Input: dimensioned drawing with shaded views. Units: mm. Origin: part minimum x, y, z. A direction names the side the tool comes from. Give positions to 0.01 mm unless a question says otherwise; leave off trailing zeros. Order: outer loops, then holes, each group sorted by start corner. A loop starts at its lowest first (then second) coordinate and runs counter-clockwise, first axis right, second up.
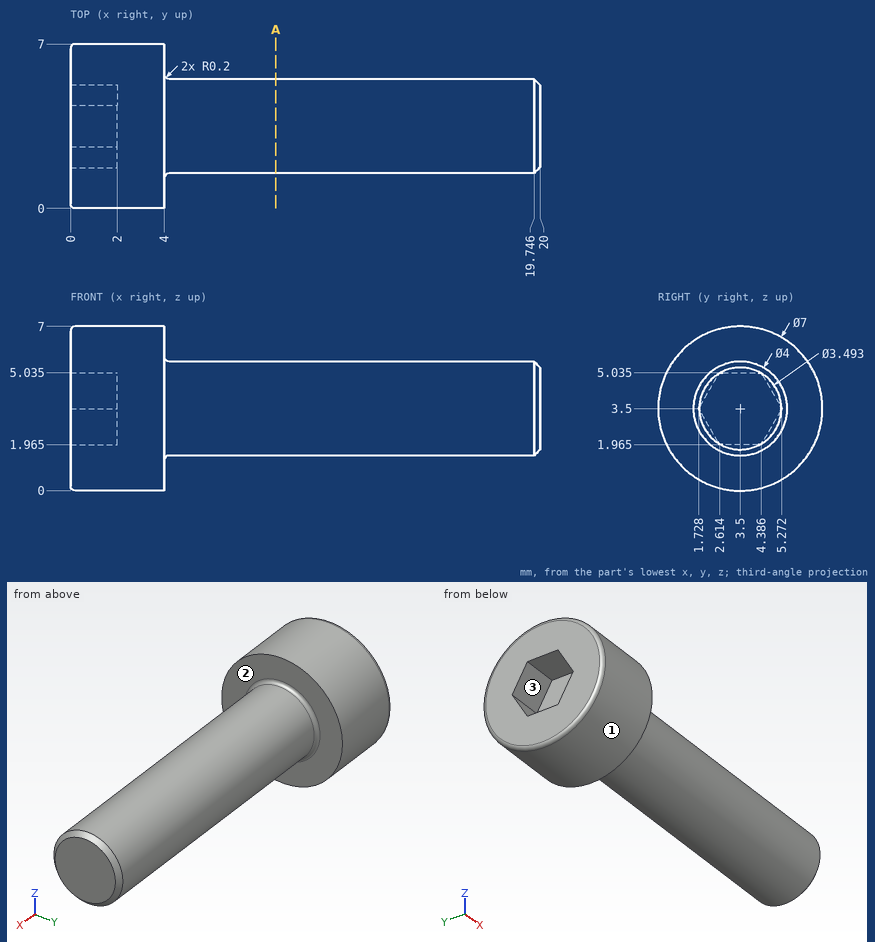
1) Pin query (flat end, axial travel): pin 1 (3 mm diameter, centred on x = 16.5, z = 6, fed in from -Y). Return the tip coordinate at first contact, or that it passes through.
Report:
pin 1: stops at y = 1.77
2) Section query A-A, the plane x = 8.75. Return the cut outline in (y, z), and give its area (3 significant figures).
Report:
outline: circle Ø4 at (3.5, 3.5)
area: 12.6 mm2
3) Material intervals for L1, parallel to X at y = 6, z = 3.25; L2, parallel to Y at x = 1.25, z = 2 (1 decimal); L3, parallel to X at y = 3.25, z = 4.5, sorted ascending.
Report:
L1: x = 0 to 4
L2: y = 0.3 to 2.6, 4.4 to 6.7
L3: x = 2 to 20
4) Reachability of the marked faces 1, 2 and 3 from +Z, -Z, +X, -X, +Y, -Y: full face, straight path, thin tool, end or side. Return the list, or none.
Report:
face 1: +X, -X
face 2: +X
face 3: -X
